Build history of the part. All positions in model axes, mm. A direction names the side the tool comes from. Round coordinates to 2 decimals unless told otherwise and drop trailing zeros. Write each loop counter-clockwise with the first axis right and the second up, starting at its lowest first coordinate (ties: lowest second). Pieces come first, ordered by that corner, then holes. Notation, with made-up numbers: M 8,4.25 L 31,4.25 A30 cw 31,39.25 Z; hole C -35,-10 d11. An arc over 180 degrees is marked long. Use a Markdown table: item, result.
from build123d import *

# Parameters (mm, degrees)
SKETCH_1_R                       = 50
EXTRUDE_1_DEPTH                  = 50
SKETCH_2_R                       = 44
CUT_EXTRUDE_1_DEPTH              = 37.5
CUT_EXTRUDE_START                = -9.5
SKETCH_3_R                       = 44
CUT_EXTRUDE_2_DEPTH              = 9.5
SKETCH_4_R                       = 14.75
SKETCH_4_R_2                     = 1.5
CUT_EXTRUDE_3_DEPTH              = 4
CUT_EXTRUDE_4_DEPTH              = 4
FILLET_1_R                       = 5
PATTERN_CIRCULAR_1_COUNT         = 5
FILLET_1_OF_PATTERN_CIRCULAR_1_R = 5
SKETCH_11_R                      = 59.165085767
CUT_EXTRUDE_8_DEPTH              = 10
SKETCH_15_R                      = 58.048743464
CUT_EXTRUDE_10_DEPTH             = 10


with BuildPart() as part:
    # 草图1 → 凸台-拉伸1 (new body)
    with BuildSketch(Plane(origin=(0, 0, 0), x_dir=(1, 0, 0), z_dir=(0, 1, 0))):
        with Locations(Location((0, 0, 0), (0, 0, 270))):
            Circle(SKETCH_1_R)
    extrude(amount=EXTRUDE_1_DEPTH)

    # 草图2 → 切除-拉伸1 (cut)
    with BuildSketch(Plane(origin=(0, 50, 0), x_dir=(1, 0, 0), z_dir=(0, 1, 0))):
        with Locations(Location((0, 0, 0), (0, 0, 270))):
            Circle(SKETCH_2_R)
    extrude(amount=-CUT_EXTRUDE_1_DEPTH, mode=Mode.SUBTRACT)

    # 草图3 → 切除-拉伸2 (cut)
    with BuildSketch(Plane.XZ.offset(CUT_EXTRUDE_START)):
        with Locations(Location((0, 0, 0), (0, 0, 90))):
            Circle(SKETCH_3_R)
    extrude(amount=CUT_EXTRUDE_2_DEPTH, mode=Mode.SUBTRACT)

    # 草图4 → 切除-拉伸3 (cut)
    with BuildSketch(Plane(origin=(0, 12.5, 0), x_dir=(1, 0, 0), z_dir=(0, 1, 0))):
        with Locations(Location((0, 0, 0), (0, 0, 270))):
            Circle(SKETCH_4_R)
        with Locations(Location((0, 17.5, 0), (0, 0, 270))):
            Circle(SKETCH_4_R_2)
        with Locations(Location((12.374368671, 12.374368671, 0), (0, 0, 270))):
            Circle(SKETCH_4_R_2)
        with Locations(Location((17.5, 0, 0), (0, 0, 270))):
            Circle(SKETCH_4_R_2)
        with Locations(Location((12.374368671, -12.374368671, 0), (0, 0, 270))):
            Circle(SKETCH_4_R_2)
        with Locations(Location((0, -17.5, 0), (0, 0, 270))):
            Circle(SKETCH_4_R_2)
        with Locations(Location((-12.374368671, -12.374368671, 0), (0, 0, 270))):
            Circle(SKETCH_4_R_2)
        with Locations(Location((-17.5, 0, 0), (0, 0, 270))):
            Circle(SKETCH_4_R_2)
        with Locations(Location((-12.374368671, 12.374368671, 0), (0, 0, 270))):
            Circle(SKETCH_4_R_2)
    extrude(amount=-CUT_EXTRUDE_3_DEPTH, mode=Mode.SUBTRACT)

    # 草图8 → 切除-拉伸4 (cut)
    with BuildSketch(Plane(origin=(0, 12.5, 0), x_dir=(1, 0, 0), z_dir=(0, 1, 0))):
        with BuildLine():
            Line((4.874773736, 39.701846066), (2.620190883, 21.33974226))
            ThreePointArc((2.620190883, 21.33974226), (9.760795744, 19.15664027), (15.724104585, 14.662964741))
            Line((15.724104585, 14.662964741), (29.254148065, 27.279934402))
            ThreePointArc((29.254148065, 27.279934402), (18.15961999, 35.640260968), (4.874773736, 39.701846066))
        make_face()
    cut_extrude_4 = extrude(amount=-CUT_EXTRUDE_4_DEPTH, mode=Mode.SUBTRACT)

    # 圆角1
    fillet_1_edges = [part.edges().sort_by_distance(p)[0] for p in [
        (29.254148065, 11, -27.279934402),
        (15.724104585, 11, -14.662964741),
        (2.620190883, 11, -21.33974226),
        (4.874773736, 11, -39.701846066),
    ]]
    fillet(fillet_1_edges, radius=FILLET_1_R)

    # 阵列(圆周)1: 切除-拉伸4 ×5 about axis
    pattern_circular_1_axis = Axis((0, 0, 0), (0, 1, 0))
    for i in range(1, PATTERN_CIRCULAR_1_COUNT):
        add(cut_extrude_4.rotate(pattern_circular_1_axis, i * 360 / PATTERN_CIRCULAR_1_COUNT), mode=Mode.SUBTRACT)

    # 圆角1 of 阵列(圆周)1
    fillet_1_of_pattern_circular_1_edges = [part.edges().sort_by_distance(p)[0] for p in [
        (-16.90473047, 11, -36.252311481),
        (-9.086292627, 11, -19.485617421),
        (-19.485617421, 11, -9.086292627),
        (-36.252311481, 11, -16.90473047),
        (-39.701846066, 11, 4.874773736),
        (-21.33974226, 11, 2.620190883),
        (-14.662964741, 11, 15.724104585),
        (-27.279934402, 11, 29.254148065),
        (-7.632359815, 11, 39.265087338),
        (-4.102393401, 11, 21.104984444),
        (10.423406835, 11, 18.804323703),
        (19.39238481, 11, 34.984788286),
        (34.984788286, 11, 19.39238481),
        (18.804323703, 11, 10.423406835),
        (21.104984444, 11, -4.102393401),
        (39.265087338, 11, -7.632359815),
    ]]
    fillet(fillet_1_of_pattern_circular_1_edges, radius=FILLET_1_OF_PATTERN_CIRCULAR_1_R)

    # 草图11 → 切除-拉伸8 (cut)
    with BuildSketch(Plane.XZ):
        Circle(SKETCH_11_R)
    extrude(amount=-CUT_EXTRUDE_8_DEPTH, mode=Mode.SUBTRACT)

    # 草图15 → 切除-拉伸10 (cut)
    with BuildSketch(Plane(origin=(0, 50, 0), x_dir=(1, 0, 0), z_dir=(0, 1, 0))):
        Circle(SKETCH_15_R)
    extrude(amount=-CUT_EXTRUDE_10_DEPTH, mode=Mode.SUBTRACT)


solid = part.part
Q1. Cut at B-B on z = 29. Give the cut face in (x, y), and give its area (3 significant figures).
Response values:
| item | result |
|---|---|
| outline | M -40.73,10 L -5.64,10 L -5.64,12.5 L -33.09,12.5 L -33.09,40 L -40.73,40 Z; M 16.07,10 L 40.73,10 L 40.73,40 L 33.09,40 L 33.09,12.5 L 16.07,12.5 Z |
| area | 570 mm2 |
Q2. Cut at A-A on x = -36.5. Give the cut face in (y, z).
Response values:
| item | result |
|---|---|
| outline | M 10,-34.17 L 40,-34.17 L 40,-24.57 L 12.5,-24.57 L 12.5,4.99 L 10,4.99 Z; M 10,16.36 L 12.5,16.36 L 12.5,24.57 L 40,24.57 L 40,34.17 L 10,34.17 Z |
Q3. Drill centre lines: L1, parallel to X at y = 11.35, z = 0; L2, parallel to X at y = 28.5, z = -0.5; L3, parallel to Y at x = -10, z = -23.5. Where is each one in solid material? Low to high.
Response values:
| item | result |
|---|---|
| L1 | x = -50 to -19, -16 to -14.75, 14.75 to 16, 19 to 21.5, 40 to 50 |
| L2 | x = -50 to -44, 44 to 50 |
| L3 | y = 10 to 12.5 |
Q4. Drop flat-ended pins along their axis: P1, Ø10, axis at x = -11.5, z = -10, coming from the +Y side; P2, Ø6, axis at y = 17, z = 23.5, coming from the -X side; P3, Ø6, axis at y = 34.5, z = 20.5, coming from the -X side. Give the stop position or say it passes through.
Response values:
| item | result |
|---|---|
| P1 | stops at y = 12.5 |
| P2 | stops at x = -45.6 |
| P3 | stops at x = -46.84 |
Q5. Cut at C-C on y = 33.25. Give the cut face in (x, z), and give its area (3 significant figures).
Response values:
| item | result |
|---|---|
| outline | C 0,0 d100; hole C 0,0 d88 |
| area | 1,770 mm2 |
Q6. Which spindle directions (+Z, -Z, +X, -X, +Y, -Y) get a long thin tool onto all of the face, cutting with end or side? Do faces 1 (the flat face through (-19, 12.5, -1)), 2 (the cylindrical face through (6.144, 11.268, 39.525)). Say none if no direction does.
Response values:
| item | result |
|---|---|
| face 1 | +Y |
| face 2 | +Y, -Y |
Q7. Cut at D-D on x = -3.5. Give the cut face in (y, z).
Response values:
| item | result |
|---|---|
| outline | M 10,-49.88 L 40,-49.88 L 40,-43.86 L 12.5,-43.86 L 12.5,-14.33 L 10,-14.33 Z; M 10,14.33 L 12.5,14.33 L 12.5,22.87 L 10,22.87 Z; M 10,39.62 L 12.5,39.62 L 12.5,43.86 L 40,43.86 L 40,49.88 L 10,49.88 Z |
